Part model, mm, in its own coordinate system. Face numbers are marked on the shaded views. A direction names the side the tool comes from. Round coordinates to 2 decimals unless told otherwise and drop trailing zeros. Loops run counter-clockwise (first coordinate to the right, second up) from the corner with the lowest first, then second, coordinate; pieces in that order, holes last. Notation, with made-up numbers: (-2.75, 55.25) -> (3.25, 55.25) arc R13 cw to (3.25, 64.25) -> close; hole circle Ø5 at (44.5, -13). An arc over 180 degrees is marked (long way). Use a Markdown table: item, result. Add a question column.
Item 1: Which spindle directions (+Z, -Z, +X, -X, +Y, -Y) get a long thin tool onto all of the face, cutting with end or side? Do the marked faces 1, 2 and 3. Say none if no direction does.
Item 2: Cut at B-B, the plane y = -47. List the corners of the cut face in (x, z) (3 decimals).
Item 3: Cut at A-A, the plane z = 6.5. List the corners of the cut face in (x, y) (3 decimals), plus the area to 3 significant figures.
Item 4: Probe line 1 (Y direction, x = 7, z = 25); line 2 (Y direction, x = 34, z = 14.5); line 3 (Z direction, x = 58.5, y = -17). List the from-to ranges inside material, lowest first. Write a range as [from, to].
Item 5: Flat gauge pins, fed straight in: pin 1 (12.5 mm diameter, centred on y = -16, z = 7.5, fed in from +X) (3 decimals); pin 2 (14 mm diameter, centred on y = -14, z = 25, fed in from -X); pin 3 (8.5 mm diameter, centred on y = 16.5, z = 23, fed in from -X) (3 decimals). Where does each tip first touch, or does it go through?
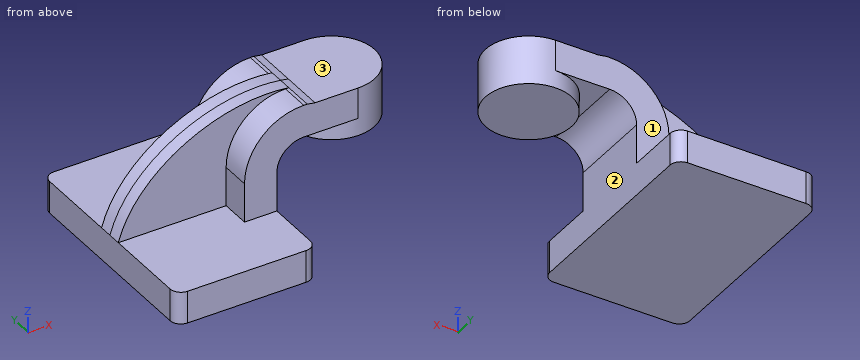
```python
from build123d import *

# Parameters (mm, degrees)
F1_DEPTH = 63.5
F0_W     = 25.4
F0_H     = 18.2524110483
F2_DEPTH = 25.4
F3_DEPTH = 7.9375
F5_R     = 6.35


with BuildPart() as f1:
    # F0 (on Front) → F1 (new body, symmetric)
    with BuildSketch(Plane.XZ):
        Polygon((-41.275, 9.525), (-41.275, -9.525), (41.275, -9.525), (41.275, 9.525), (22.225, 9.525), align=None)
    extrude(amount=F1_DEPTH, both=True)

    # F0 (on Front) → F2 (join, symmetric)
    with BuildSketch(Plane.XZ):
        with BuildLine():
            Line((22.225, 9.525), (41.275, 9.525))
            Line((41.275, 9.525), (41.275, 32.5475889517))
            ThreePointArc((41.275, 32.5475889517), (45.9246798487, 43.772909103), (57.15, 48.4225889517))
            Line((57.15, 48.4225889517), (63.746570544, 48.4225889517))
            Line((63.746570544, 48.4225889517), (63.746570544, 66.675))
            add(Edge.make_bspline(
                [(59.1752846606, 67.4725889517), (60.7111512881, 67.2512383806), (62.2357271137, 66.985690031), (63.746570544, 66.675)],
                knots=[115.2165224238, 115.2165224238, 115.2165224238, 115.2165224238, 119.5644294074, 119.5644294074, 119.5644294074, 119.5644294074], degree=3))
            Line((59.1752846606, 67.4725889517), (57.15, 67.4725889517))
            ThreePointArc((57.15, 67.4725889517), (32.4542956671, 57.2432932846), (22.225, 32.5475889517))
            Line((22.225, 32.5475889517), (22.225, 9.525))
        make_face()
        with Locations((76.446570544, 57.5487944758)):
            Rectangle(F0_W, F0_H)
    extrude(amount=F2_DEPTH, both=True)

    # F0 (on Front) → F3 (join, symmetric)
    with BuildSketch(Plane.XZ):
        with BuildLine():
            add(Edge.make_bspline(
                [(-41.275, 9.525), (-30.1520692278, 48.1675955618), (18.4758832255, 73.3382257116), (59.1752846606, 67.4725889517)],
                knots=[0, 0, 0, 0, 115.2165224238, 115.2165224238, 115.2165224238, 115.2165224238], degree=3))
            Line((-41.275, 9.525), (22.225, 9.525))
            Line((22.225, 9.525), (22.225, 32.5475889517))
            ThreePointArc((22.225, 32.5475889517), (32.4542956671, 57.2432932846), (57.15, 67.4725889517))
            Line((57.15, 67.4725889517), (59.1752846606, 67.4725889517))
        make_face()
    extrude(amount=F3_DEPTH, both=True)

    # F0 (on Front) → F4 (revolve)
    with BuildSketch(Plane.XZ):
        Polygon((114.546570544, 66.675), (89.146570544, 66.675), (89.146570544, 48.4225889517), (89.146570544, 38.1), (114.546570544, 38.1), align=None)
    revolve(axis=Axis((89.146570544, 0, 52.7862944758), (0, 0, 1)))

    # F5
    f5_edges = [f1.edges().sort_by_distance(p)[0] for p in [
        (41.275, -63.5, 0),
        (-41.275, -63.5, 0),
        (41.275, 63.5, 0),
        (-41.275, 63.5, 0),
    ]]
    fillet(f5_edges, radius=F5_R)


solid = f1.part
```
A:
| question | item | result |
|---|---|---|
| 1 | face 1 | +Z, +X, -X, +Y |
| 1 | face 2 | -Z, +X, +Y, -Y |
| 1 | face 3 | +Z, +X, +Y, -Y |
| 2 | outline | (-41.275, -9.525) -> (41.275, -9.525) -> (41.275, 9.525) -> (-41.275, 9.525) -> close |
| 3 | outline | (-41.275, -57.15) arc R6.35 ccw to (-34.925, -63.5) -> (34.925, -63.5) arc R6.35 ccw to (41.275, -57.15) -> (41.275, 57.15) arc R6.35 ccw to (34.925, 63.5) -> (-34.925, 63.5) arc R6.35 ccw to (-41.275, 57.15) -> close |
| 3 | area | 10,400 mm^2 |
| 4 | line 1 | y = [-7.94, 7.94] |
| 4 | line 2 | y = [-25.4, 25.4] |
| 4 | line 3 | z = [48.42, 67.47] |
| 5 | pin 1 | stops at x = 41.275 |
| 5 | pin 2 | stops at x = -36.44 |
| 5 | pin 3 | stops at x = 22.225 |
